Model file for the job. Use its own axes, mm. Face numbers are marked on the shaded views. Round coordinates to 2 decimals unless told otherwise and drop trailing zeros. Order: outer loops, then holes, each group sorted by start corner. A loop starts at its lowest first (then second) coordinate and runs counter-clockwise, first axis right, second up. Notation, with made-up numbers: (78, 74) -> (99, 74) arc R18 ccw to (99, 98) -> close; hole circle Ø7 at (62, -31). An arc over 180 degrees is marked (long way). Put each result on its own line as item: value. Start each with the question number.
Q1. Cut at C-C, the plane z = 9.75. List the corners of the cut face in (x, y) (3 decimals).
Q2. Cut at B-B, the plane x = 31.75. List the corners of the cut face in (y, z).
Q3. Probe L1, parallel to Y at x = 30, z = 7.25; L2, parallel to Y at x = 33.5, z = 4; L3, parallel to X at y = 7, z = 4. List the from-to ranges inside material, lowest first.
Q4. Cut at A-A, the plane z = 7.25. List the corners of the cut face in (x, y) (3 decimals), and give its area (3 significant figures).
Q5. Pull direction X, two halves, no side cores. Call the marked faces 1, 2 and 3: released by +X, released by -X, zero draft, split by the parting line, or undercut.
Autodesk Inventor part; units mm, degrees
ref_plane "YZ Plane" through (0, 0, 0) normal (1, 0, 0) x (0, 1, 0)
ref_plane "XZ Plane" through (0, 0, 0) normal (0, 1, 0) x (-1, 0, 0)
ref_plane "XY Plane" through (0, 0, 0) normal (0, 0, 1) x (1, 0, 0)
ref_plane "РабПлоскость1" through (0, 0, 0) normal (0, 0, 1) x (1, 0, 0)
sketch "Эскиз1" plane through (0, 0, 0) normal (0, 0, 1) x (1, 0, 0)
  circle A0 centre (32.975, 7.8539) radius 2
  circle A1 centre (32.975, -8.1461) radius 2
  line L0 (42.5, -30) -> (22.5, -30)
  line L1 (22.5, -30) -> (22.5, 30)
  line L2 (22.5, 30) -> (42.5, 30)
  line L3 (42.5, 30) -> (42.5, -30)
  line L4 (42.5, -30) -> (22.5, 30) construction
  line L5 (22.5, -30) -> (42.5, 30) construction
  point P0 (0, 0)
  point P1 (32.5, 0)
  point P2 (32.5, 0)
  dimension "d0" = 20
  dimension "d1" = 60
  dimension "d2" = 0
extrude "Выдавливание1" add sketch "Эскиз1" along normal blind 15
ref_plane "РабПлоскость2" through (22.5, -0.0677, -0.25) normal (1, 0, 0) x (0, -1, 0)
sketch "Эскиз2" plane through (22.5, -0.0677, -0.25) normal (1, 0, 0) x (0, -1, 0)
  circle A0 centre (-9.4216, -7.5) radius 1.2
  circle A1 centre (9.5784, -7.5) radius 1.2
  point P0 (-0.0677, -0.25)
extrude "Выдавливание2" cut sketch "Эскиз2" along normal up to surface (20 mm away)
properties part number "крепление"
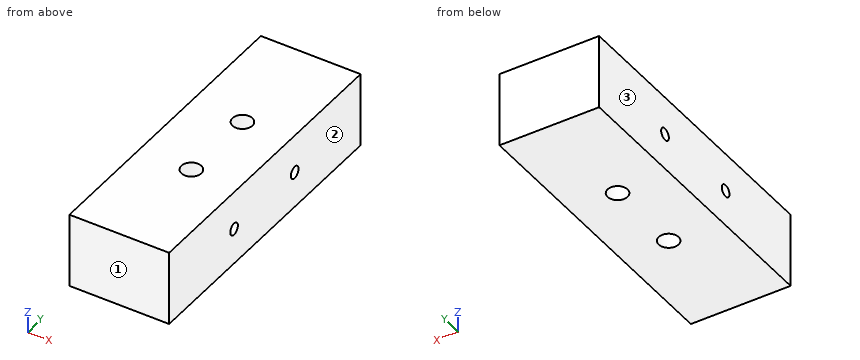
Ans:
1. outline: (22.5, -30) -> (42.5, -30) -> (42.5, 30) -> (22.5, 30) -> close; hole circle Ø4 at (32.975, -8.146); hole circle Ø4 at (32.975, 7.854)
2. outline: (-30, 0) -> (-9.73, 0) -> (-9.73, 6.05) arc R1.2 cw to (-9.73, 8.45) -> (-9.73, 15) -> (-30, 15) -> close; (-6.57, 0) -> (6.27, 0) -> (6.27, 15) -> (-6.57, 15) -> close; (9.43, 0) -> (30, 0) -> (30, 15) -> (9.43, 15) -> (9.43, 8.45) arc R1.2 cw to (9.43, 6.05) -> close
3. L1: y = -30 to -10.85, -8.45 to 8.15, 10.55 to 30
3. L2: y = -30 to -10.08, -6.22 to 5.92, 9.78 to 30
3. L3: x = 22.5 to 31.17, 34.78 to 42.5
4. outline: (22.5, -30) -> (42.5, -30) -> (42.5, -10.846) -> (22.5, -10.846) -> close; (22.5, -8.446) -> (30.998, -8.446) arc R2 cw (long way) to (34.952, -8.446) -> (42.5, -8.446) -> (42.5, 8.154) -> (34.952, 8.154) arc R2 cw (long way) to (30.998, 8.154) -> (22.5, 8.154) -> close; (22.5, 10.554) -> (42.5, 10.554) -> (42.5, 30) -> (22.5, 30) -> close
4. area: 1,090 mm^2
5. face 1: zero draft
5. face 2: released by +X
5. face 3: released by -X
